Could you check a few things on this model? Use its own coordinates, in mm. Round coordinates to 2 decimals unless told otherwise and drop trailing zeros. Write each loop counter-clockwise with the first axis right and the second up, starting at its lowest first coordinate (ties: lowest second). Pieces come first, ordered by that corner, then holes. Notation, with made-up numbers: (23.25, 53.25) - (47.25, 53.25) arc R26 ccw to (47.25, 69.25) - close; hole circle Ø7 at (-14, 60). An arc over 180 degrees is marked (long way). Put each result on its own line as item: value.
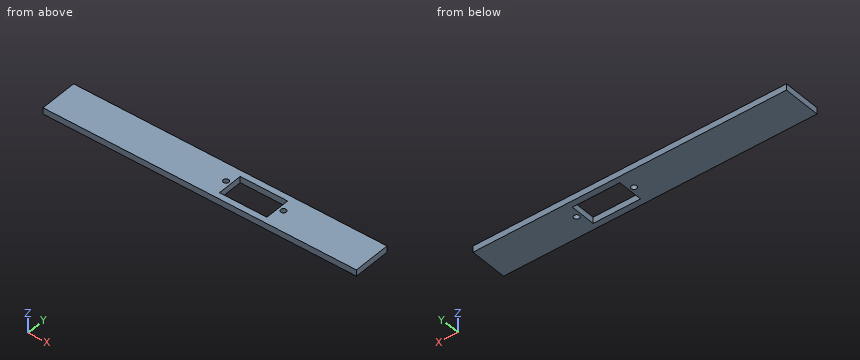
from build123d import *

# Parameters (mm, degrees)
SKETCH1_W           = 150
SKETCH1_H           = 18
BOSS_EXTRUDE1_DEPTH = 3
SKETCH2_W           = 22.7
SKETCH2_H           = 12.2
CUT_EXTRUDE1_DEPTH  = 3
SKETCH3_R           = 1.2
BOSS_EXTRUDE2_DEPTH = 3
SKETCH4_R           = 1.3
CUT_EXTRUDE2_DEPTH  = 3


with BuildPart() as part:
    # Sketch1 → Boss-Extrude1 (new body)
    with BuildSketch(Plane.XY):
        Rectangle(SKETCH1_W, SKETCH1_H)
    extrude(amount=BOSS_EXTRUDE1_DEPTH)

    # Sketch2 → Cut-Extrude1 (cut)
    with BuildSketch(Plane(origin=(0, 0, 0), x_dir=(-1, 0, 0), z_dir=(0, 0, -1))):
        with Locations((-18.45, 0)):
            Rectangle(SKETCH2_W, SKETCH2_H)
    extrude(amount=-CUT_EXTRUDE1_DEPTH, mode=Mode.SUBTRACT)

    # Sketch3 → Boss-Extrude2 (add)
    with BuildSketch(Plane.XY.offset(3)):
        with Locations((32.175, 0.1)):
            Circle(SKETCH3_R)
    extrude(amount=-BOSS_EXTRUDE2_DEPTH)

    # Sketch4 → Cut-Extrude2 (cut)
    with BuildSketch(Plane(origin=(0, 0, 0), x_dir=(-1, 0, 0), z_dir=(0, 0, -1))):
        with Locations((-32.18, 0.723190071)):
            Circle(SKETCH4_R)
        with Locations(Location((-4.72, 0.723190071, 0), (0, 0, 180))):
            Circle(SKETCH4_R)
    extrude(amount=-CUT_EXTRUDE2_DEPTH, mode=Mode.SUBTRACT)


solid = part.part
(1) Imagine slicing it at C-C, the plane z = 1.8. List the corners of the cut face in (x, y) for me.
Values found:
outline: (-75, -9) - (75, -9) - (75, 9) - (-75, 9) - close; hole circle Ø2.6 at (4.72, 0.72); hole (7.1, -6.1) - (29.8, -6.1) - (29.8, 6.1) - (7.1, 6.1) - close; hole circle Ø2.6 at (32.18, 0.72)
(2) I'm going to push a flat-ended pin straight in: pin 1 (1.5 mm diameter, centred on x = 55, y = -7, fed in from -Z). Where does the tip first touch, or does it pass through?
Values found:
pin 1: stops at z = 0
(3) Imagine slicing it at B-B, the plane x = 32.18. List the corners of the cut face in (y, z) for me, then the cut area to 3 significant figures.
Values found:
outline: (-9, 0) - (-0.58, 0) - (-0.58, 3) - (-9, 3) - close; (2.02, 0) - (9, 0) - (9, 3) - (2.02, 3) - close
area: 46.2 mm^2
(4) Please list where these lines run through material, in increasing order: probe 1 along Y at (x, z) = (7.5, 2); probe 2 along X at (y, z) = (4.75, 2.75); probe 3 along X at (y, z) = (-0.25, 2.45). Write a range as from..to.
Values found:
probe 1: y = -9..-6.1, 6.1..9
probe 2: x = -75..7.1, 29.8..75
probe 3: x = -75..3.86, 5.58..7.1, 29.8..31.32, 33.04..75
(5) Imagine slicing it at A-A, the plane y = 4. List the corners of the cut face in (x, z) for me.
Values found:
outline: (-75, 0) - (7.1, 0) - (7.1, 3) - (-75, 3) - close; (29.8, 0) - (75, 0) - (75, 3) - (29.8, 3) - close
